CAD build for the part. Positions are in the model's coordinates, mm. Face numbers are marked on the shaded views. A direction names the side the tool comes from. Coordinates: 2 decimals unless noted, no trailing zeros. Order: outer loops, then holes, each group sorted by start corner. A loop starts at its lowest first (then second) coordinate and runs counter-clockwise, first axis right, second up. Notation, with made-up numbers: M 43,81 L 51,81 A14 ccw 51,104 Z; hole C 22,74 d6. An arc over 180 degrees is marked long. Write item = value, one per line.
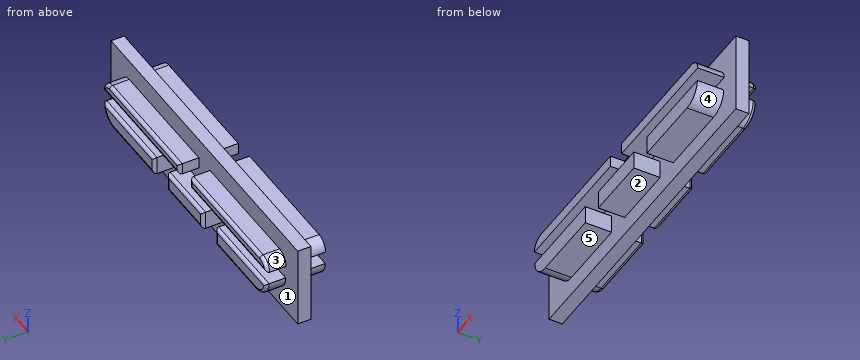
from build123d import *

# Parameters (mm, degrees)
BOSS_EXTRUDE1_DEPTH        = 2.032
BOSS_EXTRUDE1_DEPTH_BACK   = 2.54
BOSS_EXTRUDE1_2_DEPTH      = 2.032
BOSS_EXTRUDE1_2_DEPTH_BACK = 2.54
BOSS_EXTRUDE1_3_DEPTH      = 2.032
BOSS_EXTRUDE1_3_DEPTH_BACK = 2.54
SKETCH1_W                  = 4.826
SKETCH1_H                  = 1.397
BOSS_EXTRUDE1_4_DEPTH      = 2.032
BOSS_EXTRUDE1_4_DEPTH_BACK = 2.54
BOSS_EXTRUDE1_5_DEPTH      = 2.032
BOSS_EXTRUDE1_5_DEPTH_BACK = 2.54
BOSS_EXTRUDE2_DEPTH        = 0.508
BOSS_EXTRUDE2_DEPTH_BACK   = 0.508
SKETCH1_3_W                = 25.4
SKETCH1_3_H                = 6.35
SKETCH1_3_W_2              = 4.826
SKETCH1_3_H_2              = 1.397
FILLET1_R                  = 0.254


with BuildPart() as part:
    # Sketch1 → Boss-Extrude1 (new, two sides: drawn at the far end of the back side and taken through both)
    with BuildSketch(Plane(origin=(0, 3.048, 0), x_dir=(1, 0, 0), z_dir=(0, 1, 0)).offset(-BOSS_EXTRUDE1_DEPTH_BACK)):
        with BuildLine():
            Line((-9.644992793, 27.009366894), (-4.181695904, 27.009366894))
            Line((-4.181695904, 27.009366894), (-4.181695904, 25.612366894))
            Line((-4.181695904, 25.612366894), (-11.041992793, 25.612366894))
            ThreePointArc((-11.041992793, 25.612366894), (-10.632820966, 26.600195068), (-9.644992793, 27.009366894))
        make_face()
    extrude(amount=BOSS_EXTRUDE1_DEPTH + BOSS_EXTRUDE1_DEPTH_BACK)



with BuildPart() as body_2:
    # Sketch1 → Boss-Extrude1 2 (new, two sides: drawn at the far end of the back side and taken through both)
    with BuildSketch(Plane(origin=(0, 3.048, 0), x_dir=(1, 0, 0), z_dir=(0, 1, 0)).offset(-BOSS_EXTRUDE1_2_DEPTH_BACK)):
        with BuildLine():
            Line((0.776095842, 23.675616894), (10.23259664, 23.675616894))
            ThreePointArc((10.23259664, 23.675616894), (10.861214569, 23.935998966), (11.12159664, 24.564616894))
            Line((11.12159664, 24.564616894), (0.776095842, 24.564616894))
            Line((0.776095842, 24.564616894), (0.776095842, 23.675616894))
        make_face()
    extrude(amount=BOSS_EXTRUDE1_2_DEPTH + BOSS_EXTRUDE1_2_DEPTH_BACK)


with BuildPart() as body_3:
    # Sketch1 → Boss-Extrude1 3 (new, two sides: drawn at the far end of the back side and taken through both)
    with BuildSketch(Plane(origin=(0, 3.048, 0), x_dir=(1, 0, 0), z_dir=(0, 1, 0)).offset(-BOSS_EXTRUDE1_3_DEPTH_BACK)):
        with Locations((0.009304096, 26.310866894)):
            Rectangle(SKETCH1_W, SKETCH1_H)
    extrude(amount=BOSS_EXTRUDE1_3_DEPTH + BOSS_EXTRUDE1_3_DEPTH_BACK)


with BuildPart() as body_4:
    # Sketch1 → Boss-Extrude1 4 (new, two sides: drawn at the far end of the back side and taken through both)
    with BuildSketch(Plane(origin=(0, 3.048, 0), x_dir=(1, 0, 0), z_dir=(0, 1, 0)).offset(-BOSS_EXTRUDE1_4_DEPTH_BACK)):
        with BuildLine():
            Line((4.200304096, 27.009366894), (4.200304096, 25.612366894))
            Line((4.200304096, 25.612366894), (11.060600985, 25.612366894))
            ThreePointArc((11.060600985, 25.612366894), (10.651429158, 26.600195068), (9.663600985, 27.009366894))
            Line((9.663600985, 27.009366894), (4.200304096, 27.009366894))
        make_face()
    extrude(amount=BOSS_EXTRUDE1_4_DEPTH + BOSS_EXTRUDE1_4_DEPTH_BACK)


with BuildPart() as body_5:
    # Sketch1 → Boss-Extrude1 5 (new, two sides: drawn at the far end of the back side and taken through both)
    with BuildSketch(Plane(origin=(0, 3.048, 0), x_dir=(1, 0, 0), z_dir=(0, 1, 0)).offset(-BOSS_EXTRUDE1_5_DEPTH_BACK)):
        with BuildLine():
            Line((-0.75748765, 24.564616894), (-11.102988449, 24.564616894))
            ThreePointArc((-11.102988449, 24.564616894), (-10.842606377, 23.935998966), (-10.213988449, 23.675616894))
            Line((-10.213988449, 23.675616894), (-0.75748765, 23.675616894))
            Line((-0.75748765, 23.675616894), (-0.75748765, 24.564616894))
        make_face()
    extrude(amount=BOSS_EXTRUDE1_5_DEPTH + BOSS_EXTRUDE1_5_DEPTH_BACK)


with BuildPart() as part_1:
    add(part.part)

    add(body_2.part)  # Boss-Extrude2 merges body 2

    add(body_3.part)  # Boss-Extrude2 merges body 3

    add(body_4.part)  # Boss-Extrude2 merges body 4

    add(body_5.part)  # Boss-Extrude2 merges body 5
    # Sketch1_3 → Boss-Extrude2 (add, two sides: drawn at the far end of the back side and taken through both)
    with BuildSketch(Plane(origin=(0, 3.048, 0), x_dir=(1, 0, 0), z_dir=(0, 1, 0)).offset(-BOSS_EXTRUDE2_DEPTH_BACK)):
        with Locations((0.009304096, 25.273558827)):
            Rectangle(SKETCH1_3_W, SKETCH1_3_H)
        with BuildLine():
            ThreePointArc((10.23259664, 23.675616894), (10.861214569, 23.935998966), (11.12159664, 24.564616894))
            Line((11.12159664, 24.564616894), (0.776095842, 24.564616894))
            Line((0.776095842, 24.564616894), (0.776095842, 23.675616894))
            Line((0.776095842, 23.675616894), (10.23259664, 23.675616894))
        make_face(mode=Mode.SUBTRACT)
        with BuildLine():
            Line((-11.041992793, 25.612366894), (-4.181695904, 25.612366894))
            Line((-4.181695904, 25.612366894), (-4.181695904, 27.009366894))
            Line((-4.181695904, 27.009366894), (-9.644992793, 27.009366894))
            ThreePointArc((-9.644992793, 27.009366894), (-10.632820966, 26.600195068), (-11.041992793, 25.612366894))
        make_face(mode=Mode.SUBTRACT)
        with Locations((0.009304096, 26.310866894)):
            Rectangle(SKETCH1_3_W_2, SKETCH1_3_H_2, mode=Mode.SUBTRACT)
        with BuildLine():
            ThreePointArc((11.060600985, 25.612366894), (10.651429158, 26.600195068), (9.663600985, 27.009366894))
            Line((9.663600985, 27.009366894), (4.200304096, 27.009366894))
            Line((4.200304096, 27.009366894), (4.200304096, 25.612366894))
            Line((4.200304096, 25.612366894), (11.060600985, 25.612366894))
        make_face(mode=Mode.SUBTRACT)
        with BuildLine():
            Line((-0.75748765, 23.675616894), (-10.213988449, 23.675616894))
            ThreePointArc((-10.213988449, 23.675616894), (-10.842606377, 23.935998966), (-11.102988449, 24.564616894))
            Line((-11.102988449, 24.564616894), (-0.75748765, 24.564616894))
            Line((-0.75748765, 24.564616894), (-0.75748765, 23.675616894))
        make_face(mode=Mode.SUBTRACT)
    extrude(amount=BOSS_EXTRUDE2_DEPTH + BOSS_EXTRUDE2_DEPTH_BACK)

    # Fillet1
    fillet1_edges = [part_1.edges().sort_by_distance(p)[0] for p in [
        (0.009304096, 5.08, -27.009366894),
        (2.422304096, 5.08, -26.310866894),
        (-2.403695904, 5.08, -26.310866894),
        (0.009304096, 5.08, -25.612366894),
        (-10.632820966, 5.08, -26.600195068),
        (7.63045254, 5.08, -25.612366894),
        (-4.181695904, 5.08, -26.310866894),
        (10.651429158, 5.08, -26.600195068),
        (6.93195254, 5.08, -27.009366894),
        (4.200304096, 5.08, -26.310866894),
        (-6.913344348, 5.08, -27.009366894),
        (-7.611844348, 5.08, -25.612366894),
        (5.948846241, 5.08, -24.564616894),
        (0.776095842, 5.08, -24.120116894),
        (5.504346241, 5.08, -23.675616894),
        (10.861214569, 5.08, -23.935998966),
        (-0.75748765, 5.08, -24.120116894),
        (-5.485738049, 5.08, -23.675616894),
        (-10.842606377, 5.08, -23.935998966),
        (-5.930238049, 5.08, -24.564616894),
    ]]
    fillet(fillet1_edges, radius=FILLET1_R)


solid = part_1.part
(1) Slice it at B-B, the plane x = -8. Write the cut outline in (y, z), then the cut area to 3 significant figures.
Evaluation:
outline = M 0.51,-27.01 L 2.54,-27.01 L 2.54,-28.45 L 3.56,-28.45 L 3.56,-27.01 L 4.83,-27.01 A0.25 ccw 5.08,-26.76 L 5.08,-25.87 A0.25 ccw 4.83,-25.61 L 3.56,-25.61 L 3.56,-24.56 L 4.83,-24.56 A0.25 ccw 5.08,-24.31 L 5.08,-23.93 A0.25 ccw 4.83,-23.68 L 3.56,-23.68 L 3.56,-22.1 L 2.54,-22.1 L 2.54,-23.68 L 0.51,-23.68 L 0.51,-24.56 L 2.54,-24.56 L 2.54,-25.61 L 0.51,-25.61 Z
area = 14.5 mm²
(2) Wall check: line 1 (Z direction, x = -6, y = 4.45); line 2 (X direction, y = 3.65, z = -26); line 3 (Y direction, x = 11.75, z = -22.75). Give the ranges that are in metal, low to high. Write a range as from..to.
Evaluation:
line_1 = -27.01..-25.61, -24.56..-23.68
line_2 = -10.99..-4.18, -2.4..2.42, 4.2..11.01
line_3 = 2.54..3.56
(3) Slice it at C-C, the plane z = -22.75. Write the cut outline in (x, y).
Evaluation:
outline = M -12.69,2.54 L 12.71,2.54 L 12.71,3.56 L -12.69,3.56 Z
(4) Tool access for the marked faces 4 and 5: list every direction of +Z, -Z, +X, -X, +Y, -Y with a clear straight run to the whole face (end or side of a thin tool).
Evaluation:
face_4 = -Z, +X, -Y
face_5 = -Z, +X, -X, -Y
(5) Pull direction Z, two halves, no side cores. Call the marked faces 1, 2 and 3: +Z half, -Z half, draft (parallel to the pull), parting line (faces both ways), or undercut.
Evaluation:
face_1 = undercut
face_2 = -Z half
face_3 = +Z half
(6) Slice it at A-A, the plane y = 1.5. Write the cut outline in (x, z) (3 decimals).
Evaluation:
outline = M -11.103,-24.565 L -0.757,-24.565 L -0.757,-23.676 L -10.214,-23.676 A0.889 ccw Z; M -11.042,-25.612 A1.397 ccw -9.645,-27.009 L -4.182,-27.009 L -4.182,-25.612 Z; M -2.404,-27.009 L 2.422,-27.009 L 2.422,-25.612 L -2.404,-25.612 Z; M 0.776,-24.565 L 11.122,-24.565 A0.889 ccw 10.233,-23.676 L 0.776,-23.676 Z; M 4.2,-27.009 L 9.664,-27.009 A1.397 ccw 11.061,-25.612 L 4.2,-25.612 Z
(7) Pin check, flat tips, straight feed: pin 1 Ø1 at (x, y) = (-8, 4.5) entering from -Z; pin 2 Ø1 at (y, z) = (2, -24) entering from +X; pin 3 Ø1 at (x, y) = (7, 2) entering from +Z. Stop position of each tip, or through.
Evaluation:
pin_1 = -27.01
pin_2 = 11.12
pin_3 = -23.68
